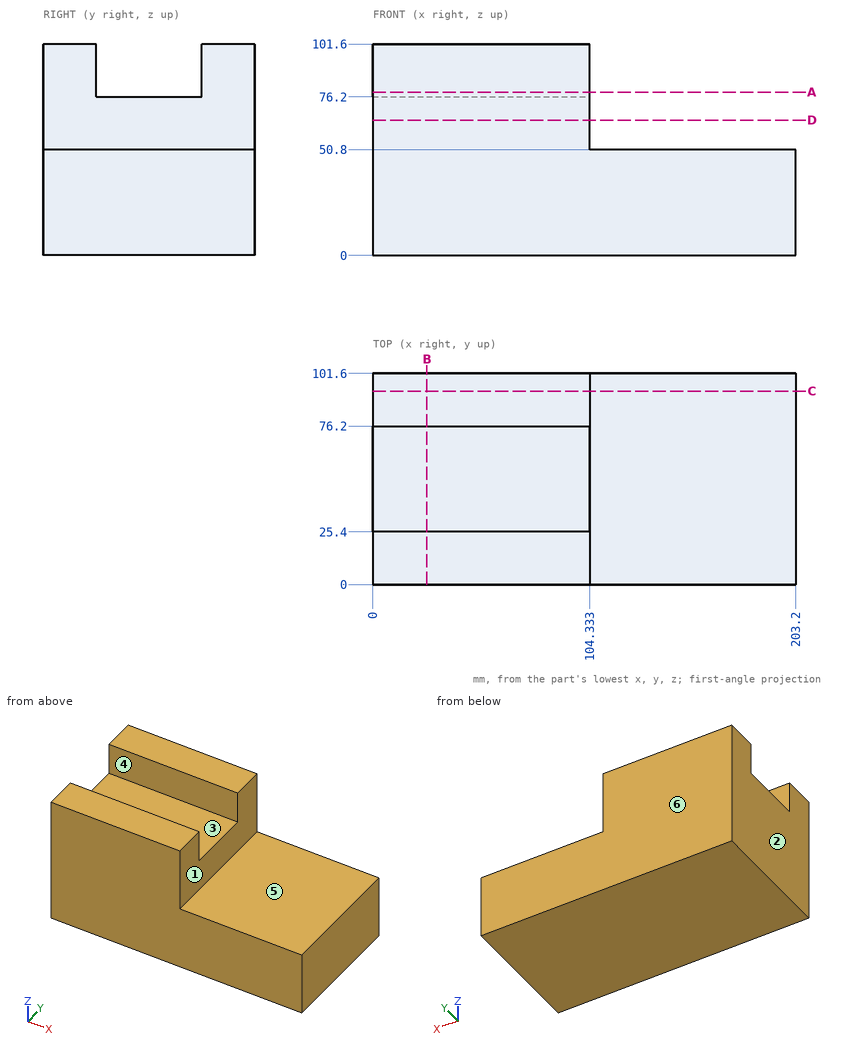
Verification items for this drawing (mm, ordinates from the low corner). A direction names the side the tool comes from. Coordinates: 2 decimals unless noted, no trailing zeros. Loops run counter-clockwise (first coordinate to the right, second up) from the corner with the lowest first, then second, coordinate; pieces in that order, holes last. Notation, with made-up numbers: (-35, 50) -> (-13, 50) arc R27 ccw to (-13, 70) -> close; hole circle Ø11 at (63.25, 82). An arc over 180 degrees is marked (long way). Put each result on its own line as item: value.
1. Gauge pin test, flat end, axial feed: P1, Ø6, axis at x = 95, y = 58, coming from the +Z side. Record the tip position at first contact, or that the pin passes through.
Result set:
P1: stops at z = 76.2
2. Thickness scan on line 1 (Y direction, x = 16, z = 81.5); line 2 (X direction, y = 24.5, z = 79.5); line 3 (Z direction, x = 110.5, y = 18). Record the ranges inside material, lowest first.
Result set:
line 1: y = 0 to 25.4, 76.2 to 101.6
line 2: x = 0 to 104.33
line 3: z = 0 to 50.8
3. Section check D-D, the plane z = 65. Record the boundary of the cut face in (x, y), then the cut area to 3 significant figures.
Result set:
outline: (0, 0) -> (104.33, 0) -> (104.33, 101.6) -> (0, 101.6) -> close
area: 10,600 mm^2
4. Section check C-C, the plane y = 93. Record the boundary of the cut face in (x, z), then the cut area to 3 significant figures.
Result set:
outline: (0, 0) -> (203.2, 0) -> (203.2, 50.8) -> (104.33, 50.8) -> (104.33, 101.6) -> (0, 101.6) -> close
area: 15,600 mm^2
5. Section check B-B, the plane x = 26. Record the boundary of the cut face in (y, z).
Result set:
outline: (0, 0) -> (101.6, 0) -> (101.6, 101.6) -> (76.2, 101.6) -> (76.2, 76.2) -> (25.4, 76.2) -> (25.4, 101.6) -> (0, 101.6) -> close
6. Tool access check on the marked faces 1 and 2. Record the directions out of +Z, -Z, +X, -X, +Y, -Y that give a thin tool (end or side, any length) a straight path to the whole face; none if there is none.
Result set:
face 1: +Z, +X, +Y, -Y
face 2: +Z, -Z, -X, +Y, -Y
7. Section check A-A, the plane z = 78.5. Record the boundary of the cut face in (x, y).
Result set:
outline: (0, 0) -> (104.33, 0) -> (104.33, 25.4) -> (0, 25.4) -> close; (0, 76.2) -> (104.33, 76.2) -> (104.33, 101.6) -> (0, 101.6) -> close
8. Mould release check, pull along Y, two halves, no side actions. Record for the marked faces 3, 4, 5 and 6: pulls with the +Y half, pulls with the -Y half, needs draft (parallel to the pull), parting line crosses it, or undercut.
Result set:
face 3: undercut
face 4: undercut
face 5: needs draft
face 6: pulls with the +Y half
